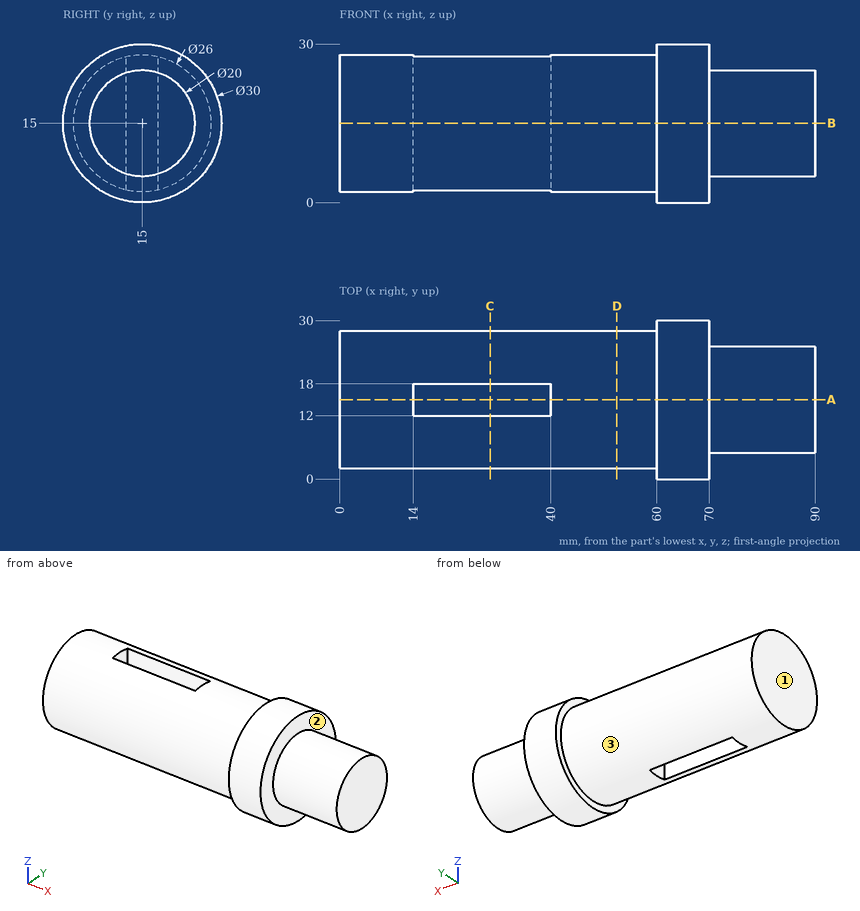
Here's the drawing with two shaded views (mm, measured from the low corner). I have some questions. A direction names the side the tool comes from. Round coordinates to 2 decimals unless told otherwise and drop trailing zeros. Loops run counter-clockwise (first coordinate to the right, second up) from the corner with the lowest first, then second, coordinate; pieces in that order, holes last.
1. If I drill on probe 1 along X at (y, z) = (14.75, 27.75); probe 2 along X at (y, z) = (12.25, 11.25); probe 3 along X at (y, z) = (24.75, 5.25), over which ranges is the centre line in solid material (lowest first)?
Answers:
probe 1: x = 0 to 14, 40 to 70
probe 2: x = 0 to 14, 40 to 90
probe 3: x = 60 to 70
2. For the marked faces 1, 2 and 3, which set-ups out of +Z, -Z, +X, -X, +Y, -Y let a thin tool reach every point of the face, with its end or its side?
Answers:
face 1: +Z, -Z, -X, +Y, -Y
face 2: +X
face 3: -X
3. Suppose I cut it at C-C, the plane x = 28.5. Please give me the cut outline in (y, z).
Answers:
outline: (12, 2.35) - (12, 27.65) arc R13 ccw to start; (18, 2.35) arc R13 ccw to (18, 27.65) - close
4. Suppose I cut it at A-A, the plane y = 15. Please give me the cut outline in (x, z), and give its area (3 significant figures).
Answers:
outline: (0, 2) - (14, 2) - (14, 28) - (0, 28) - close; (40, 2) - (60, 2) - (60, 0) - (70, 0) - (70, 5) - (90, 5) - (90, 25) - (70, 25) - (70, 30) - (60, 30) - (60, 28) - (40, 28) - close
area: 1,580 mm2
5. Will these pins go through, and if not, where does the flat tip stop? pin 1 (3 mm diameter, centred on x = 69, z = 23.5, fed in from +Y); pin 2 (10 mm diameter, centred on x = 20.5, z = 24.5, fed in from -Y); pin 3 (8 mm diameter, centred on x = 43.5, y = 5, fed in from -Z).
Answers:
pin 1: stops at y = 28.27
pin 2: stops at y = 2.8
pin 3: stops at z = 3.47
6. Suppose I cut it at D-D, the plane x = 52.5. Please give me the cut outline in (y, z).
Answers:
outline: circle Ø26 at (15, 15)
7. Suppose I cut it at B-B, the plane z = 15. Please give me the cut outline in (x, y), and give its area (3 significant figures).
Answers:
outline: (0, 2) - (60, 2) - (60, 0) - (70, 0) - (70, 5) - (90, 5) - (90, 25) - (70, 25) - (70, 30) - (60, 30) - (60, 28) - (0, 28) - close; hole (14, 12) - (40, 12) - (40, 18) - (14, 18) - close
area: 2,100 mm2
